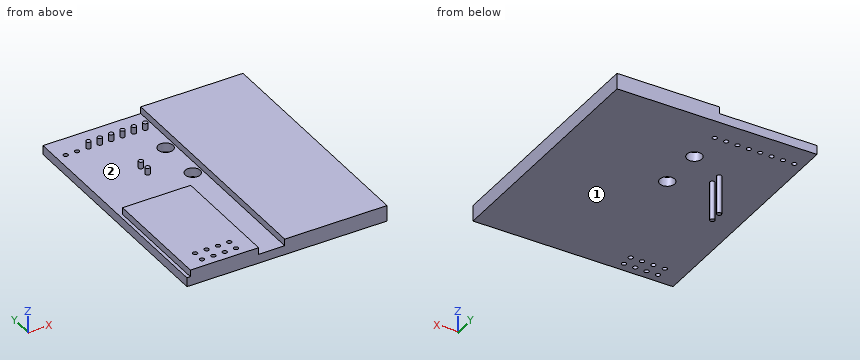
from build123d import *

# Parameters (mm, degrees)
SKETCH_W      = 44
SKETCH_H      = 53
SKETCH_R      = 1.65
SKETCH_R_2    = 0.5
PAD_DEPTH     = 2
SKETCH001_R   = 0.5
SKETCH001_W   = 22.5
SKETCH001_H   = 53
SKETCH001_W_2 = 15
SKETCH001_H_2 = 25
PAD001_DEPTH  = 2
SKETCH002_R   = 0.5
PAD002_DEPTH  = 10


with BuildPart() as part:
    # Sketch → Pad (new body)
    with BuildSketch(Plane.XY):
        with Locations((16, 26.5)):
            Rectangle(SKETCH_W, SKETCH_H)
        with Locations((13.5, 40.5)):
            Circle(SKETCH_R, mode=Mode.SUBTRACT)
        with Locations((13.5, 30.5)):
            Circle(SKETCH_R, mode=Mode.SUBTRACT)
        with Locations((1, 48)):
            Circle(SKETCH_R_2, mode=Mode.SUBTRACT)
        with Locations((3.5, 48)):
            Circle(SKETCH_R_2, mode=Mode.SUBTRACT)
        with Locations((6, 48)):
            Circle(SKETCH_R_2, mode=Mode.SUBTRACT)
        with Locations((8.5, 48)):
            Circle(SKETCH_R_2, mode=Mode.SUBTRACT)
        with Locations((11, 48)):
            Circle(SKETCH_R_2, mode=Mode.SUBTRACT)
        with Locations((13.5, 48)):
            Circle(SKETCH_R_2, mode=Mode.SUBTRACT)
        with Locations((-4, 48)):
            Circle(SKETCH_R_2, mode=Mode.SUBTRACT)
        with Locations((-1.5, 48)):
            Circle(SKETCH_R_2, mode=Mode.SUBTRACT)
        with Locations((3.5, 4.5)):
            Circle(SKETCH_R_2, mode=Mode.SUBTRACT)
        with Locations((6, 4.5)):
            Circle(SKETCH_R_2, mode=Mode.SUBTRACT)
        with Locations((-1.5, 4.5)):
            Circle(SKETCH_R_2, mode=Mode.SUBTRACT)
        with Locations((1, 4.5)):
            Circle(SKETCH_R_2, mode=Mode.SUBTRACT)
        with Locations((3.5, 2)):
            Circle(SKETCH_R_2, mode=Mode.SUBTRACT)
        with Locations((6, 2)):
            Circle(SKETCH_R_2, mode=Mode.SUBTRACT)
        with Locations((-1.5, 2)):
            Circle(SKETCH_R_2, mode=Mode.SUBTRACT)
        with Locations((1, 2)):
            Circle(SKETCH_R_2, mode=Mode.SUBTRACT)
    extrude(amount=PAD_DEPTH)

    # Sketch001 → Pad001 (join)
    with BuildSketch(Plane.XY.offset(1.5)):
        with Locations((1, 48)):
            Circle(SKETCH001_R)
        with Locations((3.5, 48)):
            Circle(SKETCH001_R)
        with Locations((6, 48)):
            Circle(SKETCH001_R)
        with Locations((8.5, 48)):
            Circle(SKETCH001_R)
        with Locations((11, 48)):
            Circle(SKETCH001_R)
        with Locations((13.5, 48)):
            Circle(SKETCH001_R)
        with Locations((6, 37.0492)):
            Circle(SKETCH001_R)
        with Locations((6, 34.5492)):
            Circle(SKETCH001_R)
        with Locations((26.75, 26.5)):
            Rectangle(SKETCH001_W, SKETCH001_H)
        with Locations((2.25, 12.5)):
            Rectangle(SKETCH001_W_2, SKETCH001_H_2)
        with Locations((3.5, 4.515131)):
            Circle(SKETCH001_R, mode=Mode.SUBTRACT)
        with Locations((6, 4.515131)):
            Circle(SKETCH001_R, mode=Mode.SUBTRACT)
        with Locations((-1.5, 4.515131)):
            Circle(SKETCH001_R, mode=Mode.SUBTRACT)
        with Locations((1, 4.515131)):
            Circle(SKETCH001_R, mode=Mode.SUBTRACT)
        with Locations((3.5, 2.015131)):
            Circle(SKETCH001_R, mode=Mode.SUBTRACT)
        with Locations((6, 2.015131)):
            Circle(SKETCH001_R, mode=Mode.SUBTRACT)
        with Locations((-1.5, 2.015131)):
            Circle(SKETCH001_R, mode=Mode.SUBTRACT)
        with Locations((1, 2.015131)):
            Circle(SKETCH001_R, mode=Mode.SUBTRACT)
    extrude(amount=PAD001_DEPTH)

    # Sketch002 → Pad002 (join)
    with BuildSketch(Plane.XY.offset(1.5)):
        with Locations((6, 37.0492)):
            Circle(SKETCH002_R)
        with Locations((6, 34.5492)):
            Circle(SKETCH002_R)
    extrude(amount=-PAD002_DEPTH)


solid = part.part
Verification items for the finished model (mm, model axes). Face numbers are marked on the shaded views. Coordinates: 2 decimals unless noted, no trailing zeros. Order: outer loops, then holes, each group sorted by start corner. A loop starts at its lowest first (then second) coordinate and runs counter-clockwise, first axis right, second up. Notation, with made-up numbers: M -25.75,47.25 L 14.25,47.25 A27 cw 14.25,84.25 Z; hole C 81,23 d4. An arc over 180 degrees is marked long. One line per item, written item: value. Start each with the question number.
Item 1: Sectioned sample at B-B (x = 25). Enter the section's corners in (y, z), then the cut area to 4 significant figures.
Item 2: Gauge pin test, flat ends, axial feed: pin 1 (1.5 mm diameter, centred on x = 2.5, y = 34.5, fed in from -Z); pin 2 (2 mm diameter, centred on x = 13.5, y = 40.5, fed in from -Z); pin 3 (0.8 mm diameter, centred on x = 13.5, y = 48, fed in from -Z); pin 4 (0.8 mm diameter, centred on y = 15.5, z = 3, fed in from -X). Record the tip position at first contact, or that the pin passes through.
Item 3: Sectioned sample at D-D (z = -5.5). Enter the section's corners in (x, y), then the cut area to 3 significant figures.
Item 4: Mould release check, pull along X, two halves, no side actions. Record for the marked faces 1 and 2: released by +X, released by -X, zero draft, split by the parting line, or undercut.
Item 5: Sectioned sample at C-C (y = 16). Enter the section's corners in (x, z), then the cut area to 3 significant figures.
Item 6: Scan lines: probe 1 along Y at (x, z) = (-1.5, 3.1); probe 2 along X at (y, z) = (4.5, 0.85); probe 3 along Y at (x, z) = (1, 0.7). Record each from-to range of solid material in increasing order.
Item 7: Sectioned sample at A-A (y = 40.5). Enter the section's corners in (x, z), then the cut area to 3 significant figures.
Conclusion:
1. outline: M 0,0 L 53,0 L 53,3.5 L 0,3.5 Z
1. area: 185.5 mm^2
2. pin 1: stops at z = 0
2. pin 2: passes through
2. pin 3: stops at z = 1.5
2. pin 4: stops at x = -5.25
3. outline: C 6,34.55 d1; C 6,37.05 d1
3. area: 1.57 mm^2
4. face 1: zero draft
4. face 2: undercut
5. outline: M -6,0 L 38,0 L 38,3.5 L 15.5,3.5 L 15.5,2 L 9.75,2 L 9.75,3.5 L -5.25,3.5 L -5.25,2 L -6,2 Z
5. area: 144 mm^2
6. probe 1: y = 0 to 1.52, 2.52 to 4.02, 5.02 to 25
6. probe 2: x = -6 to -2, -1 to 0.5, 1.5 to 3, 4 to 5.5, 6.5 to 38
6. probe 3: y = 0 to 1.5, 2.5 to 4, 5 to 47.5, 48.5 to 53
7. outline: M -6,0 L 11.85,0 L 11.85,2 L -6,2 Z; M 15.15,0 L 38,0 L 38,3.5 L 15.5,3.5 L 15.5,2 L 15.15,2 Z
7. area: 115 mm^2
